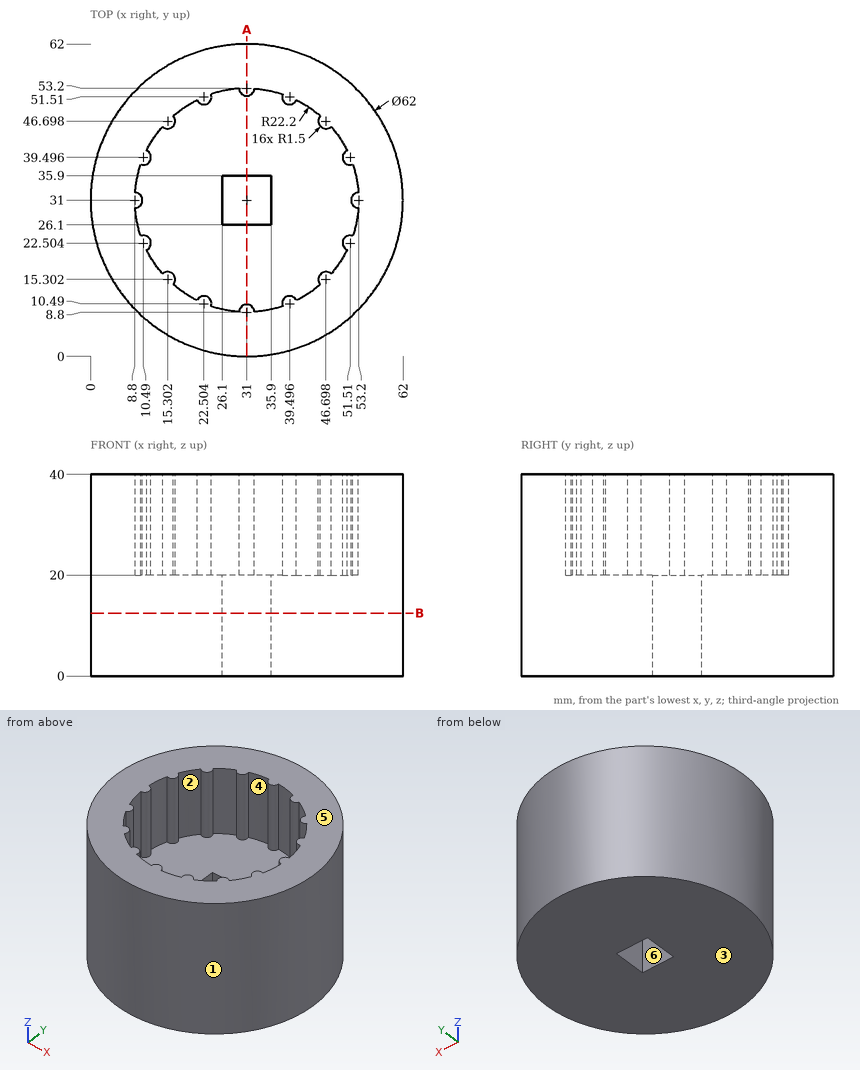
Geometry check sheet. Reference: drawing and pictorial views, mm from the part's lowest x, y, z. A direction names the side the tool comes from. Give positions to 0.01 mm unless a question says otherwise; leave off trailing zeros. Loops run counter-clockwise (first coordinate to the right, second up) from the corner with the lowest first, then second, coordinate; pieces in that order, holes last. Notation, with made-up numbers: (-14.5, 51) -> (-3.5, 51) arc R32 ccw to (-3.5, 83) -> close; hole circle Ø2 at (88.25, 14). An arc over 180 degrees is marked (long way). Answer in a Markdown table with one row per item. Add a question column.
1) Gauge pin test, flat ends, axial feed: P1, Ø3, axis at x = 32, z = 6.5, coming from the +Y side; P2, Ø12, axis at x = 55, z = 17.5, coming from the -Y side; P3, Ø12, axis at x = 55.5, z = 35.5, coming from the -Y side (1 decimal). Record the tip position at first contact, or that the pin passes through.
2) Set-up check for the marked faces 4, 5 and 6: record each of +Z, -Z, +X, -X, +Y, -Y from which the full face is reachable in a straight line by a thin tool's end or side.
3) Material ranges on probe 1 along Z at (x, y) = (41.5, 27.5); probe 2 along Y at (x, z) = (26.5, 32); probe 3 along X at (y, z) = (35, 24.5), recorded low to high. Write a range as from..to.
4) Cross-section at B-B on z = 12.5. Record the boundary of the cut face in (x, y), and give its area (3 significant figures).
5) Cross-section at A-A on x = 31. Record the boundary of the cut face in (y, z).
6) Draft check along Y on the marked faces 1, 2 and 3. Enter one of: pulls with the +Y half, pulls with the -Y half, needs draft (parallel to the pull), parting line crosses it, or undercut.
Outcome:
| question | item | result |
|---|---|---|
| 1 | P1 | stops at y = 62 |
| 1 | P2 | stops at y = 5.76 |
| 1 | P3 | stops at y = 6.1 |
| 2 | face 4 | +Z |
| 2 | face 5 | +Z, +X, -X, +Y, -Y |
| 2 | face 6 | +Z, -Z |
| 3 | probe 1 | z = 0..20 |
| 3 | probe 2 | y = 0.33..9.26, 52.74..61.67 |
| 3 | probe 3 | x = 0.26..9.16, 52.84..61.74 |
| 4 | outline | circle Ø62 at (31, 31); hole (26.1, 26.1) -> (35.9, 26.1) -> (35.9, 35.9) -> (26.1, 35.9) -> close |
| 4 | area | 2,920 mm^2 |
| 5 | outline | (0, 0) -> (26.1, 0) -> (26.1, 20) -> (10.3, 20) -> (10.3, 40) -> (0, 40) -> close; (35.9, 0) -> (62, 0) -> (62, 40) -> (51.7, 40) -> (51.7, 20) -> (35.9, 20) -> close |
| 6 | face 1 | parting line crosses it |
| 6 | face 2 | undercut |
| 6 | face 3 | needs draft |
